The listing builds one solid part. Answer for the finished solid, in the listing's coordinates (mm). Face numbers are marked on the shaded views. A direction names the side the tool comes from. Give positions to 0.01 mm unless a question says otherwise; leave off trailing zeros. Order: outer loops, then holes, each group sorted by start corner. A loop starts at its lowest first (then second) coordinate and runs counter-clockwise, first axis right, second up. Notation, with made-up numbers: (21.25, -22) - (74.25, -22) arc R24 ccw to (74.25, -6) - close; hole circle Ø3 at (-34.75, 72.5). An arc over 180 degrees is marked (long way). Write each question's results on one line, items separated by ' | '. Start each with the question number.
1. Which of the six approach directions +Z, -Z, +X, -X, +Y, -Y give full straight-line access (tool end or side, diameter ignored) to the marked faces 1 and 2?
2. Section B-B (x = 70) is taken. Give the vertices of the cut face in (y, z), and give its area (3 significant figures).
3. Section A-A (z = -28) is taken. Give the vertices of the cut face in (x, y).
4. Section D-D (z = -4) is taken. State how many separate pieces and enclosed holes the cut face has, and give its area (3 significant figures).
5. Flat-ended cylindrical pins translate along their axes: pin 1 (3 mm diameter, centred on x = 7, y = 3.5, fed in from -Z); pin 2 (3.5 mm diameter, centred on x = 70, z = -28, fed in from -Y); pin 3 (5 mm diameter, centred on x = 67.5, z = -8, fed in from +Y). Find the tip coordinate at first contact, or state that the pin passes through.
6. Find the intervals of material crossed by L1, parallel to Z at x = 82, y = 3.5; L2, parallel to Z at x = -14.5, y = 4.3; L3, parallel to X at y = 2.8, z = 14.45, in increasing order.
from build123d import *

# Parameters (mm, degrees)
BOSS_EXTRUDE1_DEPTH                                = 5.55
SKETCH2_W                                          = 39
SKETCH2_H                                          = 55
CUT_EXTRUDE1_DEPTH                                 = 1.55
FILLET1_R                                          = 8
CBORE_FOR_M2_5_PAN_HEAD_MACHINE_SCREW1_D           = 3.1
CBORE_FOR_M2_5_PAN_HEAD_MACHINE_SCREW1_CBORE_D     = 6
CBORE_FOR_M2_5_PAN_HEAD_MACHINE_SCREW1_CBORE_DEPTH = 2.1
FILLET2_R                                          = 2
CHAMFER1_SIZE                                      = 1.55
F_6_CLEARANCE_HOLE1_D                              = 4.3053


with BuildPart() as part:
    # Sketch1 → Boss-Extrude1 (new body)
    with BuildSketch(Plane(origin=(0, 0, 0), x_dir=(1, 0, 0), z_dir=(0, 1, 0))):
        Polygon((-38, -18.75), (94, -18.75), (94, 36.25), (58, 36.25), (58, 18.75), (-38, 18.75), align=None)
    extrude(amount=BOSS_EXTRUDE1_DEPTH)

    # Sketch2 → Cut-Extrude1 (cut)
    with BuildSketch(Plane(origin=(0, 5.55, 0), x_dir=(1, 0, 0), z_dir=(0, 1, 0))):
        with Locations((74.5, 8.75)):
            Rectangle(SKETCH2_W, SKETCH2_H)
    extrude(amount=-CUT_EXTRUDE1_DEPTH, mode=Mode.SUBTRACT)

    # Fillet1
    fillet1_edges = [part.edges().sort_by_distance(p)[0] for p in [
        (-38, 2.775, 18.75),
        (-38, 2.775, -18.75),
        (94, 2, 18.75),
    ]]
    fillet(fillet1_edges, radius=FILLET1_R)

    # CBORE for M2.5 Pan Head Machine Screw1 (through all)
    with Locations(Plane(origin=(0, 0, 0), x_dir=(-1, 0, 0), z_dir=(0, -1, 0))):
        with Locations((-82, 28), (-82, 4), (-70, 4), (-70, 28)):
            CounterBoreHole(CBORE_FOR_M2_5_PAN_HEAD_MACHINE_SCREW1_D / 2, CBORE_FOR_M2_5_PAN_HEAD_MACHINE_SCREW1_CBORE_D / 2, CBORE_FOR_M2_5_PAN_HEAD_MACHINE_SCREW1_CBORE_DEPTH)

    # Fillet2
    fillet2_edges = [part.edges().sort_by_distance(p)[0] for p in [
        (94, 2, -36.25),
        (58, 2, -18.75),
        (58, 2, -36.25),
    ]]
    fillet(fillet2_edges, radius=FILLET2_R)

    # Chamfer1
    chamfer1_edges = [part.edges().sort_by_distance(p)[0] for p in [
        (55, 5.55, 0),
    ]]
    chamfer(chamfer1_edges, length=CHAMFER1_SIZE - 0.0001)  # a hair under: the kernel refuses the full size

    # #6 Clearance Hole1 (through all)
    with Locations(Plane(origin=(0, 0, 0), x_dir=(-1, 0, 0), z_dir=(0, -1, 0))):
        with Locations((-32.175187039, 9.779), (-32.175187039, -9.779), (32.175187039, 9.779), (32.175187039, -9.779), (13.470384182, -14.45), (-13.470384182, -14.45), (13.470384182, 14.45), (-13.470384182, 14.45)):
            Hole(F_6_CLEARANCE_HOLE1_D / 2)


solid = part.part
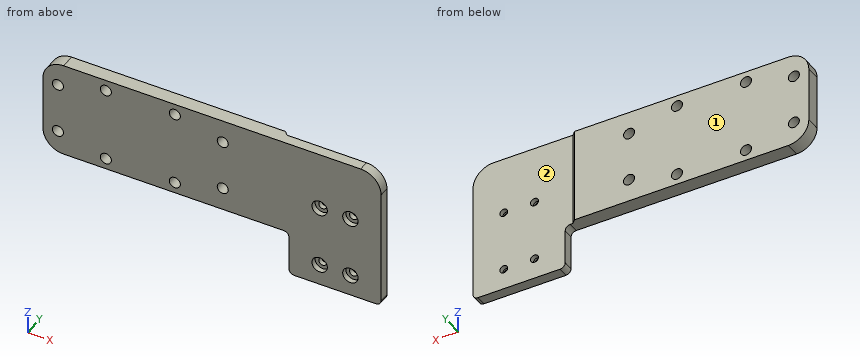
Reported:
1) face 1: +Z, -Z, +X, -X, +Y | face 2: +Z, -Z, +X, +Y
2) outline: (0, -36.25) - (4, -36.25) - (4, -29.55) - (2.1, -29.55) - (2.1, -31) - (0, -31) - close; (0, -25) - (2.1, -25) - (2.1, -26.45) - (4, -26.45) - (4, -5.55) - (2.1, -5.55) - (2.1, -7) - (0, -7) - close; (0, -1) - (2.1, -1) - (2.1, -2.45) - (4, -2.45) - (4, 18.75) - (0, 18.75) - close | area: 183 mm²
3) outline: (58, 0) - (67, 0) - (67, 2.1) - (68.45, 2.1) - (68.45, 4) - (58, 4) - close; (71.55, 2.1) - (73, 2.1) - (73, 0) - (79, 0) - (79, 2.1) - (80.45, 2.1) - (80.45, 4) - (71.55, 4) - close; (83.55, 2.1) - (85, 2.1) - (85, 0) - (94, 0) - (94, 4) - (83.55, 4) - close
4) separate pieces: 3 | enclosed holes: 0 | area: 634 mm²
5) pin 1: z = -18.75 | pin 2: y = 2.1 | pin 3: y = 4
6) L1: -36.25 to -29.55, -26.45 to -5.55, -2.45 to 18.75 | L2: -18.75 to -16.34, -12.56 to 12.56, 16.34 to 18.75 | L3: -37.09 to -15.62, -11.32 to 11.32, 15.62 to 93.09
